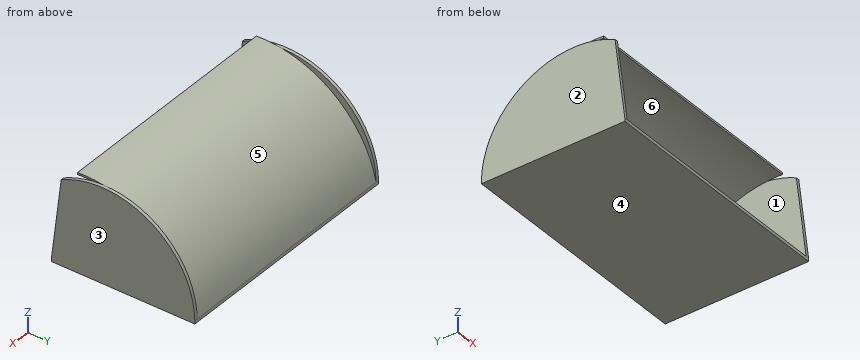
```python
from build123d import *

# Parameters (mm, degrees)
SKETCH1_W           = 186.603203036
SKETCH1_H           = 113.057286536
BOSS_EXTRUDE1_DEPTH = 2.54
BOSS_EXTRUDE2_DEPTH = 186.603203
BOSS_EXTRUDE3_DEPTH = 2.54


with BuildPart() as part:
    # Sketch1 → Boss-Extrude1 (new body)
    with BuildSketch(Plane.XY):
        Rectangle(SKETCH1_W, SKETCH1_H)
    extrude(amount=BOSS_EXTRUDE1_DEPTH)

    # Sketch2 → Boss-Extrude2 (add)
    with BuildSketch(Plane.ZY.offset(93.301601518)):
        with BuildLine():
            Line((2.54, 56.528643268), (2.54, 55.310857912))
            ThreePointArc((2.54, 55.310857912), (55.518181309, 22.042232547), (73.424493654, -37.898180421))
            Line((73.424493654, -37.898180421), (75.017810549, -37.898180421))
            ThreePointArc((75.017810549, -37.898180421), (56.529746856, 22.939984252), (2.54, 56.528643268))
        make_face()
    extrude(amount=-BOSS_EXTRUDE2_DEPTH)

    # Sketch3 → Boss-Extrude3 (add)
    with BuildSketch(Plane.ZY.offset(93.301601518)):
        with BuildLine():
            Line((2.54, 56.528643268), (0, 56.528643268))
            Line((0, 56.528643268), (0, -56.528643268))
            Line((0, -56.528643268), (2.54, -56.528643268))
            Line((2.54, -56.528643268), (66.282828168, -48.823781984))
            ThreePointArc((66.282828168, -48.823781984), (63.598341423, 21.511799087), (2.54, 56.528643268))
        make_face()
    boss_extrude3 = extrude(amount=BOSS_EXTRUDE3_DEPTH)

    # Mirror1: Boss-Extrude3 across plane
    add(boss_extrude3.mirror(Plane(origin=(0, 0, 0), x_dir=(0, 0, 1), z_dir=(1, 0, 0))))


solid = part.part
```
Geometry check sheet. Reference: the model listing, model coordinates, mm. Face numbers are marked on the shaded views. A direction names the side the tool comes from. Give positions to 0.01 mm unless a question says otherwise; leave off trailing zeros. Order: outer loops, then holes, each group sorted by start corner. A loop starts at its lowest first (then second) coordinate and runs counter-clockwise, first axis right, second up. Notation, with made-up numbers: (86.5, -27.75) -> (107.5, -27.75) arc R28 cw to (107.5, 7.25) -> close; hole circle Ø4 at (-8.5, 38.25). An arc over 180 degrees is marked (long way). Write each question's results on one line, items separated by ' | '. Start each with the question number.
(1) Gauge pin test, flat ends, axial feed: P1, Ø5, axis at x = 41.5, z = 32.5, coming from the +Y side; P2, Ø3, axis at x = 6.5, y = -36, coming from the +Z side; P3, Ø10, axis at x = -31.5, y = -27, coming from the -Z side; P4, Ø1.5, axis at x = 12, z = 55, coming from the +Y side. Record the tip position at first contact, or that the pin passes through.
(2) Sectioned sample at B-B (y = 10). Enter the section's corners in (x, z).
(3) Sectioned sample at C-C (x = 19). Enter the section's corners in (y, z).
(4) Sectioned sample at D-D (y = -42). Enter the section's corners in (x, z).
(5) Sectioned sample at A-A (z = 11). Enter the section's corners in (x, y).
(6) Access from +Z, -Z, +X, -X, +Y, -Y to the whole of each face (thin tool, end or side, straight path). Record for the marked faces 1 and 2.
(7) Mould release check, pull along Z, two halves, no side actions. Record for the marked faces 3, 4, 5 and 6: pulls with the +Z half, pulls with the -Z half, needs draft (parallel to the pull), parting line crosses it, or undercut.
(8) Scan lines: line 1 (X direction, y = 47.5, z = 5); line 2 (Z direction, x = 78, y = -32); line 3 (Z direction, x = -48, y = -47.5). Record each from-to range of solid material in increasing order.
Answer below:
1) P1: y = 46.19 | P2: z = 75.17 | P3: z = 0 | P4: y = 25.79
2) outline: (-95.84, 0) -> (95.84, 0) -> (95.84, 69.24) -> (93.3, 69.24) -> (93.3, 64.81) -> (-93.3, 64.81) -> (-93.3, 69.24) -> (-95.84, 69.24) -> close; hole (-93.3, 2.54) -> (93.3, 2.54) -> (93.3, 63.23) -> (-93.3, 63.23) -> close
3) outline: (-56.53, 0) -> (56.53, 0) -> (56.53, 2.54) arc R90.34 ccw to (-37.9, 75.02) -> (-37.9, 73.42) arc R88.82 cw to (55.31, 2.54) -> (-56.53, 2.54) -> close
4) outline: (-95.84, 0) -> (95.84, 0) -> (95.84, 69.3) -> (93.3, 69.3) -> (93.3, 2.54) -> (-93.3, 2.54) -> (-93.3, 69.3) -> (-95.84, 69.3) -> close
5) outline: (-95.84, -55.51) -> (-93.3, -55.51) -> (-93.3, 53.15) -> (93.3, 53.15) -> (93.3, -55.51) -> (95.84, -55.51) -> (95.84, 55.91) -> (93.3, 55.91) -> (93.3, 54.41) -> (-93.3, 54.41) -> (-93.3, 55.91) -> (-95.84, 55.91) -> close
6) face 1: -Y | face 2: +Z, -Z, -X, +Y, -Y
7) face 3: needs draft | face 4: pulls with the -Z half | face 5: pulls with the +Z half | face 6: undercut
8) line 1: -95.84 to -93.3, 93.3 to 95.84 | line 2: 0 to 2.54, 73.64 to 75.21 | line 3: 0 to 2.54
